from build123d import *

# Parameters (mm, degrees)
SKETCH1_R           = 5.0165
SKETCH1_R_2         = 1.778
BOSS_EXTRUDE1_DEPTH = 9.906


with BuildPart() as part:
    # Sketch1 → Boss-Extrude1 (new body)
    with BuildSketch(Plane(origin=(0, 0, 0), x_dir=(0, 0, -1), z_dir=(1, 0, 0))):
        with BuildLine():
            Line((-6.35, -34.97547742), (-6.35, 50.8))
            Line((-6.35, 50.8), (6.35, 50.8))
            Line((6.35, 50.8), (6.35, -34.97547742))
            ThreePointArc((6.35, -34.97547742), (0, -58.674000048), (-6.35, -34.97547742))
        make_face()
        with Locations((0, -45.974000048)):
            Circle(SKETCH1_R, mode=Mode.SUBTRACT)
        with Locations((-8.128, -45.974000048)):
            Circle(SKETCH1_R_2, mode=Mode.SUBTRACT)
        with Locations((0, -37.846000048)):
            Circle(SKETCH1_R_2, mode=Mode.SUBTRACT)
        with Locations((8.128, -45.974000048)):
            Circle(SKETCH1_R_2, mode=Mode.SUBTRACT)
        with Locations((0, -54.102000048)):
            Circle(SKETCH1_R_2, mode=Mode.SUBTRACT)
    extrude(amount=BOSS_EXTRUDE1_DEPTH)


solid = part.part
Geometry: final body of the model. Coordinates: model frame, mm. A direction names the side the tool comes from. Coordinates: 2 decimals unless noted, no trailing zeros. Loops run counter-clockwise (first coordinate to the right, second up) from the corner with the lowest first, then second, coordinate; pieces in that order, holes last. Notation, with made-up numbers: (1.5, 41.25) - (41.5, 41.25) arc R22 cw to (41.5, 56.25) - close; hole circle Ø4 at (-14.5, 42.5). An arc over 180 degrees is marked (long way). Put each result on its own line as item: value. Start each with the question number.
Q1. Cut plane B-B, the plane x = 4.75. Return loops of the section in (y, z).
Q2. Cut plane A-A, the plane z = 0. Return loops of the section in (x, y), and give its area (3 significant figures).
Q3. Pin query (flat end, axial travel): pin 1 Ø2 at (y, z) = (-45.974, -8.128) entering from -X; pin 2 Ø3 at (x, z) = (1.5, -7) entering from -Y; pin 3 Ø1 at (x, y) = (1.5, 0.5) entering from -Z; pin 4 Ø2 at (x, z) = (3.5, 5) entering from -Y. Return the tip coordinate at first contact, or that it passes through.
Q4. Set-up query: faces 4 (the flat face through (5, 7, 6.35)), 5 (the cylindrical face through (4.88, -47.06, -6.72)), 6 (the flat face through (5, 9, -6.35)). Return all of +Z, -Z, +X, -X, +Y, -Y with unobstructed straight access to the full face (end or side cutting, diameter ignored); none if empty.
Q5. Pull-direction query (Z, two-part tool) for faces 1 (the cylindrical face through (4.884, -55.838, 0.385)), 2 (the cylindrical face through (4.884, -58.665, -0.465)), 3 (the flat face through (9.906, -3, 0)); classes: released by +Z, released by -Z, zero draft, split by the parting line, or undercut.
Q6. Line query: line 1 (Y direction, x = 4.5, z = 0); line 2 (Y direction, x = 3, z = 1.25); line 3 (Z direction, x = 5.75, y = -31.5). Output: solid intervals per line, ascending.
Q7. Cut plane C-C, the plane y = 44. Return loops of the section in (x, z), and give its area (3 significant figures).
Filled sheet:
1. outline: (-34.98, -6.35) - (50.8, -6.35) - (50.8, 6.35) - (-34.98, 6.35) arc R12.7 ccw (long way) to start; hole circle Ø3.56 at (-54.1, 0); hole circle Ø10.03 at (-45.97, 0); hole circle Ø3.56 at (-45.97, -8.13); hole circle Ø3.56 at (-45.97, 8.13); hole circle Ø3.56 at (-37.85, 0)
2. outline: (0, -58.67) - (9.91, -58.67) - (9.91, -55.88) - (0, -55.88) - close; (0, -52.32) - (9.91, -52.32) - (9.91, -50.99) - (0, -50.99) - close; (0, -40.96) - (9.91, -40.96) - (9.91, -39.62) - (0, -39.62) - close; (0, -36.07) - (9.91, -36.07) - (9.91, 50.8) - (0, 50.8) - close
2. area: 915 mm²
3. pin 1: through
3. pin 2: y = -57.42
3. pin 3: z = -6.35
3. pin 4: y = -58.03
4. face 4: +Z, +X, -X, +Y
4. face 5: +X, -X
4. face 6: -Z, +X, -X, +Y
5. face 1: undercut
5. face 2: split by the parting line
5. face 3: zero draft
6. line 1: -58.67 to -55.88, -52.32 to -50.99, -40.96 to -39.62, -36.07 to 50.8
6. line 2: -58.61 to -55.37, -52.84 to -50.83, -41.12 to -39.11, -36.58 to 50.8
6. line 3: -6.35 to 6.35
7. outline: (0, -6.35) - (9.91, -6.35) - (9.91, 6.35) - (0, 6.35) - close
7. area: 126 mm²
